Here's how the part is built. I have some questions about the finished solid (model axes, mm). Coordinates: 2 decimals unless noted, no trailing zeros. Write each loop counter-clockwise with the first axis right and the second up, starting at its lowest first coordinate (ties: lowest second). Pieces come first, ordered by that corner, then holes. Notation, with made-up numbers: M 1.5,-8 L 52.5,-8 A20 ccw 52.5,26 Z; hole C -37,-40 d1. An arc over 180 degrees is marked long. Use a Markdown table: item, result.
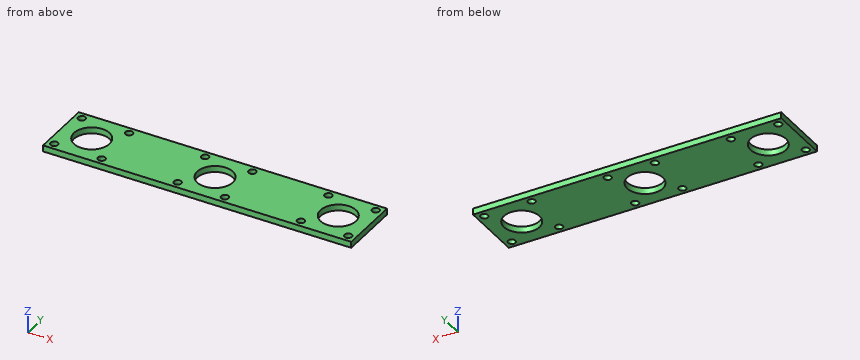
```python
from build123d import *

# Parameters (mm, degrees)
SKETCH1_W           = 127
SKETCH1_H           = 25.4
SKETCH1_R           = 7.3152
SKETCH1_R_2         = 1.524
BOSS_EXTRUDE7_DEPTH = 2.54


with BuildPart() as part:
    # Sketch1 → Boss-Extrude7 (new body)
    with BuildSketch(Plane.XY):
        Rectangle(SKETCH1_W, SKETCH1_H)
        Circle(SKETCH1_R, mode=Mode.SUBTRACT)
        with Locations((9.748400853, 9.748400853)):
            Circle(SKETCH1_R_2, mode=Mode.SUBTRACT)
        with Locations((-9.748400853, -9.748400853)):
            Circle(SKETCH1_R_2, mode=Mode.SUBTRACT)
        with Locations((9.748400853, -9.748400853)):
            Circle(SKETCH1_R_2, mode=Mode.SUBTRACT)
        with Locations((-9.748400853, 9.748400853)):
            Circle(SKETCH1_R_2, mode=Mode.SUBTRACT)
        with Locations((50.8, 0)):
            Circle(SKETCH1_R, mode=Mode.SUBTRACT)
        with Locations((60.548400853, 9.748400853)):
            Circle(SKETCH1_R_2, mode=Mode.SUBTRACT)
        with Locations((41.051599147, -9.748400853)):
            Circle(SKETCH1_R_2, mode=Mode.SUBTRACT)
        with Locations((60.548400853, -9.748400853)):
            Circle(SKETCH1_R_2, mode=Mode.SUBTRACT)
        with Locations((41.051599147, 9.748400853)):
            Circle(SKETCH1_R_2, mode=Mode.SUBTRACT)
        with Locations((-50.8, 0)):
            Circle(SKETCH1_R, mode=Mode.SUBTRACT)
        with Locations((-41.051599147, 9.748400853)):
            Circle(SKETCH1_R_2, mode=Mode.SUBTRACT)
        with Locations((-60.548400853, -9.748400853)):
            Circle(SKETCH1_R_2, mode=Mode.SUBTRACT)
        with Locations((-41.051599147, -9.748400853)):
            Circle(SKETCH1_R_2, mode=Mode.SUBTRACT)
        with Locations((-60.548400853, 9.748400853)):
            Circle(SKETCH1_R_2, mode=Mode.SUBTRACT)
    extrude(amount=BOSS_EXTRUDE7_DEPTH)


solid = part.part
```
1. I need wall thicknesses on probe 1 along X at (y, z) = (1.5, 0.1); probe 2 along Y at (x, z) = (-40.5, 1.05); probe 3 along X at (y, z) = (5.5, 0.7). Which ranges of each line are inside material? Lowest first, please.
Answers follow:
| item | result |
|---|---|
| probe 1 | x = -63.5 to -57.96, -43.64 to -7.16, 7.16 to 43.64, 57.96 to 63.5 |
| probe 2 | y = -12.7 to -11.17, -8.33 to 8.33, 11.17 to 12.7 |
| probe 3 | x = -63.5 to -55.62, -45.98 to -4.82, 4.82 to 45.98, 55.62 to 63.5 |
2. Suppose I cut it at D-D on z = 1.2. State how many separate pieces and enclosed holes the cut face has, and give its area (3 significant figures).
Answers follow:
| item | result |
|---|---|
| separate pieces | 1 |
| enclosed holes | 15 |
| area | 2,630 mm2 |
3. Suppose I cut it at B-B on x = 50.8. Write out the boundary of the cut face in (y, z).
Answers follow:
| item | result |
|---|---|
| outline | M -12.7,0 L -7.32,0 L -7.32,2.54 L -12.7,2.54 Z; M 7.32,0 L 12.7,0 L 12.7,2.54 L 7.32,2.54 Z |
4. Suppose I cut it at A-A on y = 0. Write out the boundary of the cut face in (x, z).
Answers follow:
| item | result |
|---|---|
| outline | M -63.5,0 L -58.12,0 L -58.12,2.54 L -63.5,2.54 Z; M -43.48,0 L -7.32,0 L -7.32,2.54 L -43.48,2.54 Z; M 7.32,0 L 43.48,0 L 43.48,2.54 L 7.32,2.54 Z; M 58.12,0 L 63.5,0 L 63.5,2.54 L 58.12,2.54 Z |
5. Suppose I cut it at C-C on x = 9.5. Write out the boundary of the cut face in (y, z), and give its area (3 significant figures).
Answers follow:
| item | result |
|---|---|
| outline | M -12.7,0 L -11.25,0 L -11.25,2.54 L -12.7,2.54 Z; M -8.24,0 L 8.24,0 L 8.24,2.54 L -8.24,2.54 Z; M 11.25,0 L 12.7,0 L 12.7,2.54 L 11.25,2.54 Z |
| area | 49.2 mm2 |
